from build123d import *

# Parameters (mm, degrees)
SKETCH1_W           = 40.64
SKETCH1_H           = 25.4
SKETCH1_R           = 3.175
SKETCH1_W_2         = 21.59
SKETCH1_H_2         = 19.05
BOSS_EXTRUDE1_DEPTH = 55.88
FILLET1_R           = 5.08
CHAMFER1_SIZE       = 0.254


with BuildPart() as part:
    # Sketch1 → Boss-Extrude1 (new body)
    with BuildSketch(Plane.XY):
        Rectangle(SKETCH1_W, SKETCH1_H)
        with Locations((-15.875, 5.715)):
            Circle(SKETCH1_R, mode=Mode.SUBTRACT)
        with Locations((15.875, 5.715)):
            Circle(SKETCH1_R, mode=Mode.SUBTRACT)
        with Locations((15.875, -5.715)):
            Circle(SKETCH1_R, mode=Mode.SUBTRACT)
        with Locations((-15.875, -5.715)):
            Circle(SKETCH1_R, mode=Mode.SUBTRACT)
        Rectangle(SKETCH1_W_2, SKETCH1_H_2, mode=Mode.SUBTRACT)
    extrude(amount=BOSS_EXTRUDE1_DEPTH)

    # Fillet1
    fillet1_edges = [part.edges().sort_by_distance(p)[0] for p in [
        (20.32, -12.7, 27.94),
        (-20.32, -12.7, 27.94),
        (-20.32, 12.7, 27.94),
        (20.32, 12.7, 27.94),
    ]]
    fillet(fillet1_edges, radius=FILLET1_R)

    # Chamfer1
    chamfer1_edges = [part.edges().sort_by_distance(p)[0] for p in [
        (-19.05, 5.715, 0),
        (-19.05, 5.715, 55.88),
        (12.7, 5.715, 0),
        (12.7, 5.715, 55.88),
        (12.7, -5.715, 0),
        (12.7, -5.715, 55.88),
        (-19.05, -5.715, 0),
        (-19.05, -5.715, 55.88),
        (10.795, 0, 0),
        (0, 9.525, 0),
        (-10.795, 0, 0),
        (0, -9.525, 0),
        (10.795, 0, 55.88),
        (0, 9.525, 55.88),
        (-10.795, 0, 55.88),
        (0, -9.525, 55.88),
        (0, -12.7, 0),
        (0, -12.7, 55.88),
        (20.32, 0, 0),
        (-20.32, 0, 0),
        (0, 12.7, 0),
        (-18.832102448, 11.212102448, 0),
        (18.832102448, 11.212102448, 0),
        (18.832102448, -11.212102448, 0),
        (-18.832102448, -11.212102448, 0),
        (-20.32, 0, 55.88),
        (20.32, 0, 55.88),
        (0, 12.7, 55.88),
        (-18.832102448, 11.212102448, 55.88),
        (18.832102448, 11.212102448, 55.88),
        (18.832102448, -11.212102448, 55.88),
        (-18.832102448, -11.212102448, 55.88),
    ]]
    chamfer(chamfer1_edges, length=CHAMFER1_SIZE)


solid = part.part
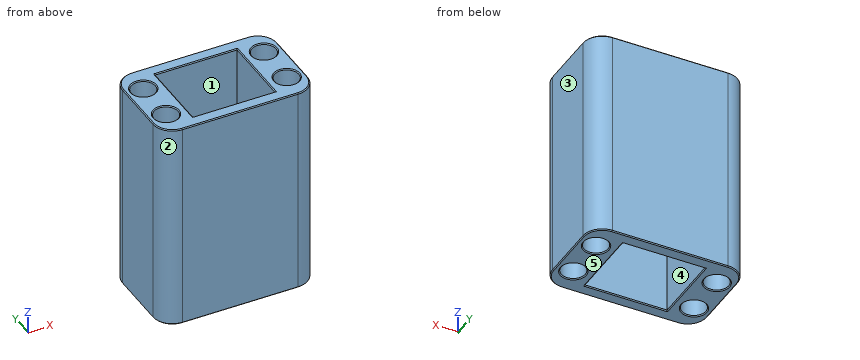
Here's how the part is built. I have some questions about the finished solid (model axes, mm). Face numbers are marked on the shaded views. A direction names the side the tool comes from. Round coordinates to 2 decimals unless told otherwise and drop trailing zeros. Loops run counter-clockwise (first coordinate to the right, second up) from the corner with the lowest first, then second, coordinate; pieces in that order, holes last. Notation, with made-up numbers: (-23.75, 31.5) -> (4.25, 31.5) arc R17 cw to (4.25, 63.5) -> close; hole circle Ø1 at (10.5, -8.5). An arc over 180 degrees is marked (long way). Write each question's results on one line, items separated by ' | '.
(1) If we section it at B-B, the plane y = -1.5: List the corners of the cut face in (x, z) for me (3 decimals).
Worked answers:
outline: (-20.32, 0.254) -> (-20.066, 0) -> (-11.049, 0) -> (-10.795, 0.254) -> (-10.795, 55.626) -> (-11.049, 55.88) -> (-20.066, 55.88) -> (-20.32, 55.626) -> close; (10.795, 0.254) -> (11.049, 0) -> (20.066, 0) -> (20.32, 0.254) -> (20.32, 55.626) -> (20.066, 55.88) -> (11.049, 55.88) -> (10.795, 55.626) -> close
(2) We'd pull the mould along X, two halves only. Please class the marked faces 3, 4 and 5: released by +X, released by -X, zero draft, split by the parting line, or undercut.
Worked answers:
face 3: released by +X | face 4: undercut | face 5: zero draft
(3) For P1, Ø4, axis at x = -15.875, y = 5.715, coming from the -Z side, with a flat end and sliding along its axis, tell me the tip position at first contact or that it passes through.
Worked answers:
P1: through
(4) If we section it at C-C, the plane z = 27.5: List the corners of the cut face in (x, y) for me (3 decimals), then the cut area to 3 significant figures.
Worked answers:
outline: (-20.32, -7.62) arc R5.08 ccw to (-15.24, -12.7) -> (15.24, -12.7) arc R5.08 ccw to (20.32, -7.62) -> (20.32, 7.62) arc R5.08 ccw to (15.24, 12.7) -> (-15.24, 12.7) arc R5.08 ccw to (-20.32, 7.62) -> close; hole circle Ø6.35 at (-15.875, -5.715); hole circle Ø6.35 at (-15.875, 5.715); hole (-10.795, -9.525) -> (10.795, -9.525) -> (10.795, 9.525) -> (-10.795, 9.525) -> close; hole circle Ø6.35 at (15.875, -5.715); hole circle Ø6.35 at (15.875, 5.715) | area: 472 mm2
(5) If we section it at A-A, the plane x = 8.5: List the corners of the cut face in (y, z) for me (3 decimals).
Worked answers:
outline: (-12.7, 0.254) -> (-12.446, 0) -> (-9.779, 0) -> (-9.525, 0.254) -> (-9.525, 55.626) -> (-9.779, 55.88) -> (-12.446, 55.88) -> (-12.7, 55.626) -> close; (9.525, 0.254) -> (9.779, 0) -> (12.446, 0) -> (12.7, 0.254) -> (12.7, 55.626) -> (12.446, 55.88) -> (9.779, 55.88) -> (9.525, 55.626) -> close
(6) If we section it at D-D, the plane x = 14: Give the number of separate pieces and of enclosed holes in the cut face, then the cut area to 3 significant figures.
Worked answers:
separate pieces: 3 | enclosed holes: 0 | area: 846 mm2
(7) For the marked faces 1 and 2, which set-ups out of +Z, -Z, +X, -X, +Y, -Y let a thin tool reach every point of the face, with its end or its side?
Worked answers:
face 1: +Z, -Z | face 2: +Z, -Z, -X, -Y
(8) If I drill on L1, parallel to Y at x = 8.5, z = 38 (3 decimals); L2, parallel to X at y = -5, z = 7 (3 decimals); L3, parallel to Y at x = 14.5, z = 10, over which ranges is the centre line in solid material (lowest first)?
Worked answers:
L1: -12.7 to -9.525, 9.525 to 12.7 | L2: -20.32 to -18.968, -12.782 to -10.795, 10.795 to 12.782, 18.968 to 20.32 | L3: -12.7 to -8.58, -2.85 to 2.85, 8.58 to 12.7
